```python
from build123d import *

# Parameters (mm, degrees)
BOSS_EXTRUDE2_DEPTH      = 33.02
BOSS_EXTRUDE2_DEPTH_BACK = 33.02
SKETCH5_W                = 50.93744157
SKETCH5_H                = 46.03648482
CUT_EXTRUDE2_DEPTH       = 71.12
SKETCH9_R                = 12.7
SKETCH9_R_2              = 9.525
BOSS_EXTRUDE3_DEPTH      = 7.62
CUT_EXTRUDE3_REACH       = 86.659
SKETCH10_R               = 0.75
CUT_EXTRUDE4_REACH       = 112.716
SKETCH11_W               = 20.066
SKETCH11_H               = 41.148


with BuildPart() as part:
    # Sketch3 → Boss-Extrude2 (new, two sides: drawn at the far end of the back side and taken through both)
    with BuildSketch(Plane.XY.offset(-BOSS_EXTRUDE2_DEPTH_BACK)):
        with BuildLine():
            Line((-31.917133282, 0), (18.882866718, 0))
            Line((18.882866718, 0), (18.882866718, 50.8))
            Line((18.882866718, 50.8), (16.643514063, 63.5))
            ThreePointArc((16.643514063, 63.5), (-6.517133282, 82.934090645), (-29.677780627, 63.5))
            Line((-29.677780627, 63.5), (-31.917133282, 50.8))
            Line((-31.917133282, 50.8), (-31.917133282, 0))
        make_face()
    extrude(amount=BOSS_EXTRUDE2_DEPTH + BOSS_EXTRUDE2_DEPTH_BACK)

    # Sketch5 → Cut-Extrude2 (cut)
    with BuildSketch(Plane(origin=(0, 82.934090645, 0), x_dir=(1, 0, 0), z_dir=(0, 1, 0))):
        with Locations((-6.517133282, 0)):
            Rectangle(SKETCH5_W, SKETCH5_H)
    extrude(amount=-CUT_EXTRUDE2_DEPTH, mode=Mode.SUBTRACT)

    # Sketch9 → Boss-Extrude3 (add)
    with BuildSketch(Plane.XZ):
        with Locations(Location((-6.517133282, 0, 0), (0, 0, 180))):
            Circle(SKETCH9_R)
        with Locations(Location((-6.517133282, 0, 0), (0, 0, 180))):
            Circle(SKETCH9_R_2, mode=Mode.SUBTRACT)
    extrude(amount=BOSS_EXTRUDE3_DEPTH)

    # Sketch10 → Cut-Extrude3 (cut, up to next)
    with BuildSketch(Plane(origin=(0, 11.814090645, 0), x_dir=(1, 0, 0), z_dir=(0, 1, 0)), mode=Mode.PRIVATE) as cut_extrude3_sk1:
        with Locations(Location((-3.214362801, -6.862339772, 0), (0, 0, 270))):
            Circle(SKETCH10_R)
    cut_extrude3_tool1 = extrude(cut_extrude3_sk1.sketch, amount=-CUT_EXTRUDE3_REACH, mode=Mode.PRIVATE) & part.part
    # Sketch10 → Cut-Extrude3 (cut, up to next)
    with BuildSketch(Plane(origin=(0, 11.814090645, 0), x_dir=(1, 0, 0), z_dir=(0, 1, 0)), mode=Mode.PRIVATE) as cut_extrude3_sk2:
        with Locations(Location((-6.211501931, -6.993324637, 0), (0, 0, 270))):
            Circle(SKETCH10_R)
    cut_extrude3_tool2 = extrude(cut_extrude3_sk2.sketch, amount=-CUT_EXTRUDE3_REACH, mode=Mode.PRIVATE) & part.part
    # Sketch10 → Cut-Extrude3 (cut, up to next)
    with BuildSketch(Plane(origin=(0, 11.814090645, 0), x_dir=(1, 0, 0), z_dir=(0, 1, 0)), mode=Mode.PRIVATE) as cut_extrude3_sk3:
        with Locations(Location((-9.208641061, -7.124309502, 0), (0, 0, 270))):
            Circle(SKETCH10_R)
    cut_extrude3_tool3 = extrude(cut_extrude3_sk3.sketch, amount=-CUT_EXTRUDE3_REACH, mode=Mode.PRIVATE) & part.part
    # Sketch10 → Cut-Extrude3 (cut, up to next)
    with BuildSketch(Plane(origin=(0, 11.814090645, 0), x_dir=(1, 0, 0), z_dir=(0, 1, 0)), mode=Mode.PRIVATE) as cut_extrude3_sk4:
        with Locations(Location((-13.379473054, -3.302770481, 0), (0, 0, 270))):
            Circle(SKETCH10_R)
    cut_extrude3_tool4 = extrude(cut_extrude3_sk4.sketch, amount=-CUT_EXTRUDE3_REACH, mode=Mode.PRIVATE) & part.part
    # Sketch10 → Cut-Extrude3 (cut, up to next)
    with BuildSketch(Plane(origin=(0, 11.814090645, 0), x_dir=(1, 0, 0), z_dir=(0, 1, 0)), mode=Mode.PRIVATE) as cut_extrude3_sk5:
        with Locations(Location((-13.510457919, -0.305631351, 0), (0, 0, 270))):
            Circle(SKETCH10_R)
    cut_extrude3_tool5 = extrude(cut_extrude3_sk5.sketch, amount=-CUT_EXTRUDE3_REACH, mode=Mode.PRIVATE) & part.part
    # Sketch10 → Cut-Extrude3 (cut, up to next)
    with BuildSketch(Plane(origin=(0, 11.814090645, 0), x_dir=(1, 0, 0), z_dir=(0, 1, 0)), mode=Mode.PRIVATE) as cut_extrude3_sk6:
        with Locations(Location((-13.641442784, 2.691507779, 0), (0, 0, 270))):
            Circle(SKETCH10_R)
    cut_extrude3_tool6 = extrude(cut_extrude3_sk6.sketch, amount=-CUT_EXTRUDE3_REACH, mode=Mode.PRIVATE) & part.part
    # Sketch10 → Cut-Extrude3 (cut, up to next)
    with BuildSketch(Plane(origin=(0, 11.814090645, 0), x_dir=(1, 0, 0), z_dir=(0, 1, 0)), mode=Mode.PRIVATE) as cut_extrude3_sk7:
        with Locations(Location((0.60717622, -2.691507779, 0), (0, 0, 270))):
            Circle(SKETCH10_R)
    cut_extrude3_tool7 = extrude(cut_extrude3_sk7.sketch, amount=-CUT_EXTRUDE3_REACH, mode=Mode.PRIVATE) & part.part
    # Sketch10 → Cut-Extrude3 (cut, up to next)
    with BuildSketch(Plane(origin=(0, 11.814090645, 0), x_dir=(1, 0, 0), z_dir=(0, 1, 0)), mode=Mode.PRIVATE) as cut_extrude3_sk8:
        with Locations(Location((0.476191355, 0.305631351, 0), (0, 0, 270))):
            Circle(SKETCH10_R)
    cut_extrude3_tool8 = extrude(cut_extrude3_sk8.sketch, amount=-CUT_EXTRUDE3_REACH, mode=Mode.PRIVATE) & part.part
    # Sketch10 → Cut-Extrude3 (cut, up to next)
    with BuildSketch(Plane(origin=(0, 11.814090645, 0), x_dir=(1, 0, 0), z_dir=(0, 1, 0)), mode=Mode.PRIVATE) as cut_extrude3_sk9:
        with Locations(Location((0.34520649, 3.302770481, 0), (0, 0, 270))):
            Circle(SKETCH10_R)
    cut_extrude3_tool9 = extrude(cut_extrude3_sk9.sketch, amount=-CUT_EXTRUDE3_REACH, mode=Mode.PRIVATE) & part.part
    # Sketch10 → Cut-Extrude3 (cut, up to next)
    with BuildSketch(Plane(origin=(0, 11.814090645, 0), x_dir=(1, 0, 0), z_dir=(0, 1, 0)), mode=Mode.PRIVATE) as cut_extrude3_sk10:
        with Locations(Location((-3.825625503, 7.124309502, 0), (0, 0, 270))):
            Circle(SKETCH10_R)
    cut_extrude3_tool10 = extrude(cut_extrude3_sk10.sketch, amount=-CUT_EXTRUDE3_REACH, mode=Mode.PRIVATE) & part.part
    # Sketch10 → Cut-Extrude3 (cut, up to next)
    with BuildSketch(Plane(origin=(0, 11.814090645, 0), x_dir=(1, 0, 0), z_dir=(0, 1, 0)), mode=Mode.PRIVATE) as cut_extrude3_sk11:
        with Locations(Location((-6.822764633, 6.993324637, 0), (0, 0, 270))):
            Circle(SKETCH10_R)
    cut_extrude3_tool11 = extrude(cut_extrude3_sk11.sketch, amount=-CUT_EXTRUDE3_REACH, mode=Mode.PRIVATE) & part.part
    # Sketch10 → Cut-Extrude3 (cut, up to next)
    with BuildSketch(Plane(origin=(0, 11.814090645, 0), x_dir=(1, 0, 0), z_dir=(0, 1, 0)), mode=Mode.PRIVATE) as cut_extrude3_sk12:
        with Locations(Location((-9.819903763, 6.862339772, 0), (0, 0, 270))):
            Circle(SKETCH10_R)
    cut_extrude3_tool12 = extrude(cut_extrude3_sk12.sketch, amount=-CUT_EXTRUDE3_REACH, mode=Mode.PRIVATE) & part.part
    add(cut_extrude3_tool1.solids().sort_by_distance((-3.214363, 11.814091, 6.86234))[0], mode=Mode.SUBTRACT)
    add(cut_extrude3_tool2.solids().sort_by_distance((-6.211502, 11.814091, 6.993325))[0], mode=Mode.SUBTRACT)
    add(cut_extrude3_tool3.solids().sort_by_distance((-9.208641, 11.814091, 7.12431))[0], mode=Mode.SUBTRACT)
    add(cut_extrude3_tool4.solids().sort_by_distance((-13.379473, 11.814091, 3.30277))[0], mode=Mode.SUBTRACT)
    add(cut_extrude3_tool5.solids().sort_by_distance((-13.510458, 11.814091, 0.305631))[0], mode=Mode.SUBTRACT)
    add(cut_extrude3_tool6.solids().sort_by_distance((-13.641443, 11.814091, -2.691508))[0], mode=Mode.SUBTRACT)
    add(cut_extrude3_tool7.solids().sort_by_distance((0.607176, 11.814091, 2.691508))[0], mode=Mode.SUBTRACT)
    add(cut_extrude3_tool8.solids().sort_by_distance((0.476191, 11.814091, -0.305631))[0], mode=Mode.SUBTRACT)
    add(cut_extrude3_tool9.solids().sort_by_distance((0.345206, 11.814091, -3.30277))[0], mode=Mode.SUBTRACT)
    add(cut_extrude3_tool10.solids().sort_by_distance((-3.825626, 11.814091, -7.12431))[0], mode=Mode.SUBTRACT)
    add(cut_extrude3_tool11.solids().sort_by_distance((-6.822765, 11.814091, -6.993325))[0], mode=Mode.SUBTRACT)
    add(cut_extrude3_tool12.solids().sort_by_distance((-9.819904, 11.814091, -6.86234))[0], mode=Mode.SUBTRACT)

    # Sketch11 → Cut-Extrude4 (cut, up to next)
    with BuildSketch(Plane.XY.offset(33.02), mode=Mode.PRIVATE) as cut_extrude4_sk1:
        with Locations((-6.517133282, 39.412411)):
            Rectangle(SKETCH11_W, SKETCH11_H)
    cut_extrude4_tool1 = extrude(cut_extrude4_sk1.sketch, amount=-CUT_EXTRUDE4_REACH, mode=Mode.PRIVATE) & part.part
    add(cut_extrude4_tool1.solids().sort_by_distance((-6.517133, 39.412411, 33.02))[0], mode=Mode.SUBTRACT)


solid = part.part
```
Geometry check sheet. Reference: the model listing, model coordinates, mm. A direction names the side the tool comes from. Give positions to 0.01 mm unless a question says otherwise; leave off trailing zeros. Loops run counter-clockwise (first coordinate to the right, second up) from the corner with the lowest first, then second, coordinate; pieces in that order, holes last. Notation, with made-up numbers: (-4, 39) - (4, 39) arc R27 cw to (4, 66) - close; hole circle Ø3 at (25, -11). An arc over 180 degrees is marked (long way). Use CSV: the item, a comma, the result in double quotes. Start each with the question number.
Q1. Release check for a two-part mould opening along X. For faces 4 (the face through (-4.45, -3.76, 9.3)), 5 (the face through (-7, 48, -23.018)), 6 (the face through (-16.55, 39, 28)), 7 (the face through (-31.917, 9, 0)) record: +X half, -X half, draft (parallel to the pull), parting line (faces both ways), or undercut.
Q2. Section check B-B, the plane z = -21. Record the cut outline in (x, y), and give its area (3 significant figures).
Q3. Section check A-A, the plane y = 35. Record the cut outline in (x, z), and give its area (3 significant figures).
Q4. Scan lines: probe 1 along X at (y, z) = (31, 30); probe 2 along Z at (x, y) = (-22.5, 61); probe 3 along Y at (x, z) = (-14, -20). Record each from-to range of solid material in increasing order. Write a range as from..to.
Q5. Section check C-C, the plane x = -23. Record the cut outline in (y, z), and give its area (3 significant figures).
Q6. Access from +Z, -Z, +X, -X, +Y, -Y to the whole of each face (thin tool, end or side, straight path). Record for faces 1 (the face through (3.516, 39, 28)), 2 (the face through (-7, 11.814, 0)), 3 (the face through (-7, 0, 0)).
Q7. Go/stop test with flat-tipped pins: pin 1 Ø6 at (x, z) = (-13.5, -9.5) entering from +Y; pin 2 Ø0.9 at (x, z) = (-13.51, 0.31) entering from +Y; pin 3 Ø2.5 at (x, z) = (-6.82, -6.99) entering from -Y; pin 4 Ø1 at (x, y) = (-12, 23.5) entering from +Z. Record where each tip stops, or that it passes through.
Findings below:
1,face 4,"undercut"
1,face 5,"draft"
1,face 6,"undercut"
1,face 7,"-X half"
2,outline,"(-31.92, 0) - (18.88, 0) - (18.88, 11.81) - (-31.92, 11.81) - close"
2,area,"600 mm^2"
3,outline,"(-31.92, -33.02) - (18.88, -33.02) - (18.88, -23.02) - (-31.92, -23.02) - close; (-31.92, 23.02) - (-16.55, 23.02) - (-16.55, 33.02) - (-31.92, 33.02) - close; (3.52, 23.02) - (18.88, 23.02) - (18.88, 33.02) - (3.52, 33.02) - close"
3,area,"815 mm^2"
4,probe 1,"x = -31.92..-16.55, 3.52..18.88"
4,probe 2,"z = -33.02..-23.02, 23.02..33.02"
4,probe 3,"y = 0..11.81"
5,outline,"(0, -33.02) - (76.19, -33.02) - (76.19, -23.02) - (11.81, -23.02) - (11.81, 23.02) - (76.19, 23.02) - (76.19, 33.02) - (0, 33.02) - close"
5,area,"2,070 mm^2"
6,face 1,"+Z"
6,face 2,"+X, -X, +Y"
6,face 3,"-Y"
7,pin 1,"stops at y = 11.81"
7,pin 2,"passes through"
7,pin 3,"stops at y = 0"
7,pin 4,"stops at z = -23.02"
